Design review of the part built by this model. Coordinates are the model's own, in mm. A direction names the side the tool comes from. Give positions to 0.01 mm unless a question says otherwise; leave off trailing zeros. Write each loop counter-clockwise with the first axis right and the second up, starting at its lowest first coordinate (ties: lowest second). Pieces come first, ordered by that corner, then holes. Notation, with made-up numbers: (24, 8) - (66, 8) arc R14 cw to (66, 20) - close; hole circle Ø3 at (-23.5, 5.5). An arc over 180 degrees is marked (long way). Use a Markdown table: item, result. Add a question column.
```python
from build123d import *

# Parameters (mm, degrees)
EXTRUDE_2_DEPTH = 15


with BuildPart() as part:
    # 草圖1 → 填料-伸長2 (new body)
    with BuildSketch(Plane.XY):
        with BuildLine():
            Line((20, -0.85915493), (20, 3.860018002))
            Line((20, 3.860018002), (23.543805166, 3.860018002))
            ThreePointArc((23.543805166, 3.860018002), (55.409150332, -4.326684577), (79.382262386, -26.85915493))
            Line((79.382262386, -26.85915493), (89.382262386, -26.85915493))
            Line((89.382262386, -26.85915493), (89.382262386, -30.85915493))
            Line((89.382262386, -30.85915493), (79.382262386, -30.85915493))
            ThreePointArc((79.382262386, -30.85915493), (54.166103207, -10.987798363), (24, 0))
            Line((24, 0), (24, -3.85915493))
            Line((24, -3.85915493), (-24, -3.85915493))
            Line((-24, -3.85915493), (-24, 0))
            ThreePointArc((-24, 0), (-54.166103207, -10.987798363), (-79.382262386, -30.85915493))
            Line((-79.382262386, -30.85915493), (-89.382262386, -30.85915493))
            Line((-89.382262386, -30.85915493), (-89.382262386, -26.85915493))
            Line((-89.382262386, -26.85915493), (-79.382262386, -26.85915493))
            ThreePointArc((-79.382262386, -26.85915493), (-55.409150332, -4.326684577), (-23.543805166, 3.860018002))
            Line((-23.543805166, 3.860018002), (-20, 3.860018002))
            Line((-20, 3.860018002), (-20, -0.85915493))
            Line((-20, -0.85915493), (20, -0.85915493))
        make_face()
    extrude(amount=EXTRUDE_2_DEPTH)


solid = part.part
```
(1) For line 1 along Y through (x, z) = (7.5, 7); line 2 along X through (y, z) = (-21, 2.25); line 3 along X through (y, z) = (-29, 1.25), list the stretches that pass through material, from the lowest coordinate up.
(2) Tool access review of faces 4 (the face through (-53.77, -10.77, 7.4)), 5 (the face through (84, -26.859, 7)), 6 (the face through (0, -0.859, 7)), 7 (the face through (-84, -30.859, 7)): name each direction out of +Z, -Z, +X, -X, +Y, -Y from which nothing blocks a thin tool from reaching the whole face with its end or side.
(3) Add section D-D (y = -9.5). State the section outline as (x, z) points.
(4) Add section A-A (z = 11.5). State the section outline as (x, y) points, and give its area (3 significant figures).
(5) Add section B-B (y = -19). State the section outline as (x, z) points.
(6) Add section C-C (x = -6). State the section outline as (y, z) points, and give its area (3 significant figures).
(7) Insertion check: pin 1 (3 mm diameter, centred on x = 71, z = 2.5, fed in from +Y); pin 2 (3 mm diameter, centred on x = -83, z = 4.5, fed in from +Y); pin 3 (6 mm diameter, centred on x = 61.5, y = -16, fed in from +Z); pin 4 (1.2 mm diameter, centred on y = -2.5, z = 7.5, fed in from +X). Each pin has a flat end and moves straight along its axis. Give the tip position at first contact, or say it passes through.
(8) Mouldability with a two-part tool opening along X and no side actions: class faces 1 (the face through (89.382, -29, 7)), 2 (the face through (0, -3, 0)), 3 (the face through (20, 1, 7)) as +X half, -X half, draft (parallel to the pull), parting line (faces both ways), or undercut.
Answers follow:
| question | item | result |
|---|---|---|
| 1 | line 1 | -3.86 to -0.86 |
| 1 | line 2 | -75.21 to -68.91, 68.91 to 75.21 |
| 1 | line 3 | -89.38 to -77.63, 77.63 to 89.38 |
| 2 | face 4 | +Z, -Z, -Y |
| 2 | face 5 | +Z, -Z, +X, +Y |
| 2 | face 6 | +Z, -Z, +Y |
| 2 | face 7 | +Z, -Z, +X, -X, -Y |
| 3 | outline | (-63.39, 0) - (-51.4, 0) - (-51.4, 15) - (-63.39, 15) - close; (51.4, 0) - (63.39, 0) - (63.39, 15) - (51.4, 15) - close |
| 4 | outline | (-89.38, -30.86) - (-79.38, -30.86) arc R101.35 cw to (-24, 0) - (-24, -3.86) - (24, -3.86) - (24, 0) arc R101.35 cw to (79.38, -30.86) - (89.38, -30.86) - (89.38, -26.86) - (79.38, -26.86) arc R66.11 ccw to (23.54, 3.86) - (20, 3.86) - (20, -0.86) - (-20, -0.86) - (-20, 3.86) - (-23.54, 3.86) arc R66.11 ccw to (-79.38, -26.86) - (-89.38, -26.86) - close |
| 4 | area | 956 mm^2 |
| 5 | outline | (-73.54, 0) - (-66.38, 0) - (-66.38, 15) - (-73.54, 15) - close; (66.38, 0) - (73.54, 0) - (73.54, 15) - (66.38, 15) - close |
| 6 | outline | (-3.86, 0) - (-0.86, 0) - (-0.86, 15) - (-3.86, 15) - close |
| 6 | area | 45.0 mm^2 |
| 7 | pin 1 | y = -14.73 |
| 7 | pin 2 | y = -26.86 |
| 7 | pin 3 | z = 15 |
| 7 | pin 4 | x = 53.07 |
| 8 | face 1 | +X half |
| 8 | face 2 | draft |
| 8 | face 3 | undercut |
